Source: CAD feature listing. Evaluate the final solid. Frame: model axes, mm. A direction names the side the tool comes from. Round coordinates to 2 decimals unless told otherwise and drop trailing zeros. Loops run counter-clockwise (first coordinate to the right, second up) from the corner with the lowest first, then second, coordinate; pieces in that order, holes last. Notation, with made-up numbers: (33, 79) - (46, 79) arc R24 ccw to (46, 90) - close; hole circle Ø3 at (20.5, 80). An arc over 180 degrees is marked (long way). One line per question, with ' | ' between items. Start each with the question number.
1. Access query for faces 3 (the flat face through (-1, 6.675, 1)), 4 (the flat face through (-1, 1, 3)). Directions: +Z, -Z, +X, -X, +Y, -Y. A direction counts if a zero-diameter tool reaches every point of the face in a straight line with its end or side. Return the directions, or none.
2. Cut plane C-C (z = 0.6). Return loops of the section in (x, y).
3. Cut plane D-D (y = 7.25). Return loops of the section in (x, z).
4. Cut plane B-B (y = -2.75). Return loops of the section in (x, z).
5. Mould query, pull axis X, two halves, no side actions, for faces 1 (the flat face through (-1, -5.677, 1)), 2 (the flat face through (-1, 1, 0)). Classes: pulls with the +X half, pulls with the -X half, needs draft (parallel to the pull), parting line crosses it, or undercut.
6. Ray query, line 1 (X direction, y = -4.5, z = 2.95); line 2 (X direction, y = -4, z = 0.75); line 3 (Y direction, x = 6.5, z = 2.1). Return the intervals inside material, ascending.
7. Pin query (flat end, axial travel): pin 1 (1.5 mm diameter, centred on x = 2.5, z = 2.5, fed in from -Y); pin 2 (1 mm diameter, centred on x = -5.5, z = 2, fed in from -Y); pin 3 (6.5 mm diameter, centred on x = -8.5, y = 0.5, fed in from +Z); pin 4 (1.5 mm diameter, centred on y = 4.5, z = 1, fed in from -X). Return the tip coordinate at first contact, or that it passes through.
8. Cut plane A-A (x = -8.5). Return loops of the section in (y, z), then the cut area to 3 significant figures.
```python
from build123d import *

# Parameters (mm, degrees)
F0_R     = 5.5
F1_DEPTH = 3


with BuildPart() as f1:
    # F0 (on Top) → F1 (new body)
    with BuildSketch(Plane.XY):
        with BuildLine():
            ThreePointArc((-0.99853, 0.499257), (-1.858995, 3.987319), (-4.24295, 6.675019))
            ThreePointArc((-4.24295, 6.675019), (-15.99853, 0.499257), (-4.24295, -5.676504))
            ThreePointArc((-4.24295, -5.676504), (-1.858995, -2.988804), (-0.99853, 0.499257))
        make_face()
        with Locations((-8.49853, 0.499257)):
            Circle(F0_R, mode=Mode.SUBTRACT)
        with BuildLine():
            Line((2.245889, 6.675019), (-4.24295, 6.675019))
            ThreePointArc((-4.24295, 6.675019), (-1.858995, 3.987319), (-0.99853, 0.499257))
            ThreePointArc((-0.99853, 0.499257), (-0.138066, 3.987319), (2.245889, 6.675019))
        make_face()
        with BuildLine():
            ThreePointArc((2.245889, -5.676504), (-0.138066, -2.988804), (-0.99853, 0.499257))
            ThreePointArc((-0.99853, 0.499257), (-1.858995, -2.988804), (-4.24295, -5.676504))
            Line((-4.24295, -5.676504), (2.245889, -5.676504))
        make_face()
        with BuildLine():
            ThreePointArc((14.00147, 0.499257), (9.989531, 7.138793), (2.245889, 6.675019))
            ThreePointArc((2.245889, 6.675019), (-0.138066, 3.987319), (-0.99853, 0.499257))
            ThreePointArc((-0.99853, 0.499257), (-0.138066, -2.988804), (2.245889, -5.676504))
            ThreePointArc((2.245889, -5.676504), (9.989531, -6.140278), (14.00147, 0.499257))
        make_face()
        with Locations((6.50147, 0.499257)):
            Circle(F0_R, mode=Mode.SUBTRACT)
    extrude(amount=F1_DEPTH)


solid = f1.part
```
Answers follow:
1) face 3: +Z, -Z, +Y | face 4: +Z, +X, -X, +Y, -Y
2) outline: (-4.24, -5.68) - (2.25, -5.68) arc R7.5 ccw (long way) to (2.25, 6.68) - (-4.24, 6.68) arc R7.5 ccw (long way) to start; hole circle Ø11 at (-8.5, 0.5); hole circle Ø11 at (6.5, 0.5)
3) outline: (-11.77, 0) - (-5.23, 0) - (-5.23, 3) - (-11.77, 3) - close; (3.23, 0) - (9.77, 0) - (9.77, 3) - (3.23, 3) - close
4) outline: (-15.26, 0) - (-12.94, 0) - (-12.94, 3) - (-15.26, 3) - close; (-4.06, 0) - (2.06, 0) - (2.06, 3) - (-4.06, 3) - close; (10.94, 0) - (13.26, 0) - (13.26, 3) - (10.94, 3) - close
5) face 1: undercut | face 2: needs draft
6) line 1: x = -14.09 to -10.79, -6.21 to 4.21, 8.79 to 12.09 | line 2: x = -14.5 to -11.66, -5.34 to 3.34, 9.66 to 12.5 | line 3: y = -7 to -5, 6 to 8
7) pin 1: stops at y = -6.26 | pin 2: stops at y = -6.57 | pin 3: passes through | pin 4: stops at x = -15.26
8) outline: (-7, 0) - (-5, 0) - (-5, 3) - (-7, 3) - close; (6, 0) - (8, 0) - (8, 3) - (6, 3) - close | area: 12.0 mm2
